from build123d import *

# Parameters (mm, degrees)
F0_R     = 4
F1_DEPTH = 352
F2_R     = 5
F3_R     = 2


with BuildPart() as f1:
    # F0 (on Top) → F1 (new body)
    with BuildSketch(Plane.XY):
        Polygon((20, 4), (20, 20), (4, 20), (4, 10), (-4, 10), (-4, 20), (-20, 20), (-20, 4), (-10, 4), (-10, -4), (-20, -4), (-20, -20), (-4, -20), (-4, -10), (4, -10), (4, -20), (20, -20), (20, -4), (10, -4), (10, 4), align=None)
        Circle(F0_R, mode=Mode.SUBTRACT)
    extrude(amount=F1_DEPTH)

    # F2
    f2_edges = [f1.edges().sort_by_distance(p)[0] for p in [
        (-20, 20, 176),
        (-20, -20, 176),
        (20, 20, 176),
        (20, -20, 176),
    ]]
    fillet(f2_edges, radius=F2_R)

    # F3
    f3_edges = [f1.edges().sort_by_distance(p)[0] for p in [
        (-4, 20, 176),
        (4, 20, 176),
        (20, 4, 176),
        (20, -4, 176),
        (4, -20, 176),
        (-4, -20, 176),
        (-20, -4, 176),
        (-20, 4, 176),
    ]]
    fillet(f3_edges, radius=F3_R)


solid = f1.part
Input: part model. Units: mm. Frame: model coordinates. A direction names the side the tool comes from. Coordinates: 2 decimals unless noted, no trailing zeros. Loops run counter-clockwise (first coordinate to the right, second up) from the corner with the lowest first, then second, coordinate; pieces in that order, holes last. Notation, with made-up numbers: (-38.5, 53) - (16.5, 53) arc R20 cw to (16.5, 83) - close; hole circle Ø10 at (66, 35.25). An arc over 180 degrees is marked (long way). Answer in a Markdown table with one row per item. Add a question column.
Item 1: Mould query, pull axis Y, two halves, no side actions, for faces 1 (the flat face through (20, 10, 174)), 2 (the cylindrical face through (-0.867, -3.905, 173.536)), 3 (the flat face through (10, -20, 174)), 4 (the flat face through (11, 20, 174)). Classes: released by +Y, released by -Y, zero draft, split by the parting line, or undercut.
Item 2: Line query: line 1 along Y through (x, z) = (0, 137.5); line 2 along X through (y, z) = (0.5, 90.5); line 3 along Y through (x, z) = (13.5, 336). Output: solid intervals per line, ascending. Write a range as [from, to].
Item 3: Contact query for flat-ended pins moving along their axis: P1, Ø10.5, axis at x = 0, y = 0, coming from the -Z side; P2, Ø9, axis at x = -0.5, z = 190.5, coming from the -Y side; P3, Ø2, axis at y = 0.5, z = 170, coming from the +X side; P4, Ø4, axis at y = -3, z = 201, coming from the +X side. Output: stop coordinate, or through.
Item 4: Access query for faces 5 (the flat face through (0, -10, 174)), 6 (the flat face through (-5, 0, 352)), 7 (the flat face through (14, 4, 174)), 8 (the flat face through (0, 10, 174)), 9 (the flat face through (-14, -4, 174)). Directions: +Z, -Z, +X, -X, +Y, -Y. A direction counts if a zero-diameter tool reaches every point of the face in a straight line with its end or side. Return the directions, or none.
Item 5: Section query A-A on x = 0. Return the cut outline in (y, z), then the cut area to 3 significant figures.
Recorded:
| question | item | result |
|---|---|---|
| 1 | face 1 | zero draft |
| 1 | face 2 | undercut |
| 1 | face 3 | released by -Y |
| 1 | face 4 | released by +Y |
| 2 | line 1 | [-10, -4], [4, 10] |
| 2 | line 2 | [-10, -3.97], [3.97, 10] |
| 2 | line 3 | [-20, -4], [4, 20] |
| 3 | P1 | z = 0 |
| 3 | P2 | y = -19.73 |
| 3 | P3 | x = 10 |
| 3 | P4 | x = 19.73 |
| 4 | face 5 | +Z, -Z, -Y |
| 4 | face 6 | +Z, +X, -X, +Y, -Y |
| 4 | face 7 | +Z, -Z, +X |
| 4 | face 8 | +Z, -Z, +Y |
| 4 | face 9 | +Z, -Z, -X |
| 5 | outline | (-10, 0) - (-4, 0) - (-4, 352) - (-10, 352) - close; (4, 0) - (10, 0) - (10, 352) - (4, 352) - close |
| 5 | area | 4,220 mm^2 |
